Autodesk Inventor part; units mm, degrees
ref_plane "YZ Plane" through (0, 0, 0) normal (1, 0, 0) x (0, 1, 0)
ref_plane "XZ Plane" through (0, 0, 0) normal (0, 1, 0) x (-1, 0, 0)
ref_plane "XY Plane" through (0, 0, 0) normal (0, 0, 1) x (1, 0, 0)
sketch "Sketch1" plane through (0, 0, 0) normal (0, 0, 1) x (1, 0, 0)
  circle A0 centre (0, 0) radius 11.9062
  dimension "d0" = 23.8125
extrude "Extrusion1" add sketch "Sketch1" along normal blind 41.275
sketch "Sketch2" plane through (0, 0, 41.275) normal (0, 0, 1) x (1, 0, 0)
  circle A0 centre (0, 0) radius 12.7
  dimension "d3" = 25.4
extrude "Extrusion2" add sketch "Sketch2" against normal blind 23.8125
sketch "Sketch3" plane through (0, 0, 41.275) normal (0, 0, 1) x (1, 0, 0)
  line L0 (-3.6662, 6.35) -> (3.6662, 6.35)
  line L1 (3.6662, 6.35) -> (7.3323, 0)
  line L2 (7.3323, 0) -> (3.6662, -6.35)
  line L3 (3.6662, -6.35) -> (-3.6662, -6.35)
  line L4 (-3.6662, -6.35) -> (-7.3323, 0)
  line L5 (-7.3323, 0) -> (-3.6662, 6.35)
  point P0 (0, 0)
  dimension "d6" = 12.7
  dimension "d7" = 12.7
  dimension "d8" = 12.7
  dimension "d9" = 120
  dimension "d10" = 120
  dimension "d11" = 6.35
  dimension "d12" = 6.35
  dimension "d13" = 6.35
extrude "Extrusion3" cut sketch "Sketch3" against normal blind 50.8
sketch "Sketch4" plane through (0, 0, 41.275) normal (0, 0, 1) x (1, 0, 0)
  line L0 (-7.3323, 0) -> (-3.6662, 6.35)
  line L1 (-3.6662, 6.35) -> (3.6662, 6.35)
  line L2 (3.6662, 6.35) -> (7.3323, 0)
  line L3 (7.3323, 0) -> (3.6662, -6.35)
  line L4 (3.6662, -6.35) -> (-3.6662, -6.35)
  line L5 (-3.6662, -6.35) -> (-7.3323, 0)
  circle A0 centre (0, 0) radius 12.7
  line L6 (0, 12.7) -> (0, 15.875) construction
  line L7 (0, 12.7) -> (3.175, 12.7) construction
  line L8 (0, 0) -> (1.9867, 12.5436) construction
  circle A1 centre (0, 0) radius 12.7 construction
  line L9 (0, 0) -> (12.7, 0) construction
  line L10 (0, 0) -> (-1.9867, 12.5436) construction
  line L11 (0, 0) -> (12.7, 0) construction
  line L12 (0, 15.875) -> (0.7937, 15.875) construction
  line L13 (0, 15.875) -> (0.7937, 15.875) construction
  line L14 (0, 15.875) -> (-0.7937, 15.875) construction
  line L15 (0, 15.875) -> (0.7937, 15.875) construction
  line L16 (-1.9867, 12.5436) -> (-0.7937, 15.875)
  line L17 (-0.7937, 15.875) -> (0.7937, 15.875)
  line L18 (0.7937, 15.875) -> (1.9867, 12.5436)
  line L19 (-1.9867, 12.5436) -> (1.9867, 12.5436)
  line L20 (-6.35, 10.9985) -> (-7.9375, 13.7482) construction
  line L21 (-6.35, 10.9985) -> (-3.6004, 12.586) construction
  line L22 (0, 0) -> (-4.5513, 11.8565) construction
  line L23 (0, 0) -> (-7.9924, 9.8698) construction
  line L24 (-7.9375, 13.7482) -> (-7.2501, 14.145) construction
  line L25 (-7.9375, 13.7482) -> (-7.2501, 14.145) construction
  line L26 (-7.9375, 13.7482) -> (-8.6249, 13.3513) construction
  line L27 (-7.9375, 13.7482) -> (-7.2501, 14.145) construction
  line L28 (-7.9924, 9.8698) -> (-8.6249, 13.3513)
  line L29 (-8.6249, 13.3513) -> (-7.2501, 14.145)
  line L30 (-7.2501, 14.145) -> (-4.5513, 11.8565)
  line L31 (-7.9924, 9.8698) -> (-4.5513, 11.8565)
  line L32 (-10.9985, 6.35) -> (-13.7482, 7.9375) construction
  line L33 (-10.9985, 6.35) -> (-9.411, 9.0996) construction
  line L34 (0, 0) -> (-9.8698, 7.9924) construction
  line L35 (0, 0) -> (-11.8565, 4.5513) construction
  line L36 (-13.7482, 7.9375) -> (-13.3513, 8.6249) construction
  line L37 (-13.7482, 7.9375) -> (-13.3513, 8.6249) construction
  line L38 (-13.7482, 7.9375) -> (-14.145, 7.2501) construction
  line L39 (-13.7482, 7.9375) -> (-13.3513, 8.6249) construction
  line L40 (-11.8565, 4.5513) -> (-14.145, 7.2501)
  line L41 (-14.145, 7.2501) -> (-13.3513, 8.6249)
  line L42 (-13.3513, 8.6249) -> (-9.8698, 7.9924)
  line L43 (-11.8565, 4.5513) -> (-9.8698, 7.9924)
  line L44 (-12.7, 0) -> (-15.875, 0) construction
  line L45 (-12.7, 0) -> (-12.7, 3.175) construction
  line L46 (0, 0) -> (-12.5436, 1.9867) construction
  line L47 (0, 0) -> (-12.5436, -1.9867) construction
  line L48 (-15.875, 0) -> (-15.875, 0.7938) construction
  line L49 (-15.875, 0) -> (-15.875, 0.7938) construction
  line L50 (-15.875, 0) -> (-15.875, -0.7937) construction
  line L51 (-15.875, 0) -> (-15.875, 0.7938) construction
  line L52 (-12.5436, -1.9867) -> (-15.875, -0.7937)
  line L53 (-15.875, -0.7937) -> (-15.875, 0.7938)
  line L54 (-15.875, 0.7938) -> (-12.5436, 1.9867)
  line L55 (-12.5436, -1.9867) -> (-12.5436, 1.9867)
  line L56 (-10.9985, -6.35) -> (-13.7482, -7.9375) construction
  line L57 (-10.9985, -6.35) -> (-12.586, -3.6004) construction
  line L58 (0, 0) -> (-11.8565, -4.5513) construction
  line L59 (0, 0) -> (-9.8698, -7.9924) construction
  line L60 (-13.7482, -7.9375) -> (-14.145, -7.2501) construction
  line L61 (-13.7482, -7.9375) -> (-14.145, -7.2501) construction
  line L62 (-13.7482, -7.9375) -> (-13.3513, -8.6249) construction
  line L63 (-13.7482, -7.9375) -> (-14.145, -7.2501) construction
  line L64 (-9.8698, -7.9924) -> (-13.3513, -8.6249)
  line L65 (-13.3513, -8.6249) -> (-14.145, -7.2501)
  line L66 (-14.145, -7.2501) -> (-11.8565, -4.5513)
  line L67 (-9.8698, -7.9924) -> (-11.8565, -4.5513)
  line L68 (-6.35, -10.9985) -> (-7.9375, -13.7482) construction
  line L69 (-6.35, -10.9985) -> (-9.0996, -9.411) construction
  line L70 (0, 0) -> (-7.9924, -9.8698) construction
  line L71 (0, 0) -> (-4.5513, -11.8565) construction
  line L72 (-7.9375, -13.7482) -> (-8.6249, -13.3513) construction
  line L73 (-7.9375, -13.7482) -> (-8.6249, -13.3513) construction
  line L74 (-7.9375, -13.7482) -> (-7.2501, -14.145) construction
  line L75 (-7.9375, -13.7482) -> (-8.6249, -13.3513) construction
  line L76 (-4.5513, -11.8565) -> (-7.2501, -14.145)
  line L77 (-7.2501, -14.145) -> (-8.6249, -13.3513)
  line L78 (-8.6249, -13.3513) -> (-7.9924, -9.8698)
  line L79 (-4.5513, -11.8565) -> (-7.9924, -9.8698)
  line L80 (0, -12.7) -> (0, -15.875) construction
  line L81 (0, -12.7) -> (-3.175, -12.7) construction
  line L82 (0, 0) -> (-1.9867, -12.5436) construction
  line L83 (0, 0) -> (1.9867, -12.5436) construction
  line L84 (0, -15.875) -> (-0.7938, -15.875) construction
  line L85 (0, -15.875) -> (-0.7938, -15.875) construction
  line L86 (0, -15.875) -> (0.7937, -15.875) construction
  line L87 (0, -15.875) -> (-0.7938, -15.875) construction
  line L88 (1.9867, -12.5436) -> (0.7937, -15.875)
  line L89 (0.7937, -15.875) -> (-0.7938, -15.875)
  line L90 (-0.7938, -15.875) -> (-1.9867, -12.5436)
  line L91 (1.9867, -12.5436) -> (-1.9867, -12.5436)
  line L92 (6.35, -10.9985) -> (7.9375, -13.7482) construction
  line L93 (6.35, -10.9985) -> (3.6004, -12.586) construction
  line L94 (0, 0) -> (4.5513, -11.8565) construction
  line L95 (0, 0) -> (7.9924, -9.8698) construction
  line L96 (7.9375, -13.7482) -> (7.2501, -14.145) construction
  line L97 (7.9375, -13.7482) -> (7.2501, -14.145) construction
  line L98 (7.9375, -13.7482) -> (8.6249, -13.3513) construction
  line L99 (7.9375, -13.7482) -> (7.2501, -14.145) construction
  line L100 (7.9924, -9.8698) -> (8.6249, -13.3513)
  line L101 (8.6249, -13.3513) -> (7.2501, -14.145)
  line L102 (7.2501, -14.145) -> (4.5513, -11.8565)
  line L103 (7.9924, -9.8698) -> (4.5513, -11.8565)
  line L104 (10.9985, -6.35) -> (13.7482, -7.9375) construction
  line L105 (10.9985, -6.35) -> (9.411, -9.0996) construction
  line L106 (0, 0) -> (9.8698, -7.9924) construction
  line L107 (0, 0) -> (11.8565, -4.5513) construction
  line L108 (13.7482, -7.9375) -> (13.3513, -8.6249) construction
  line L109 (13.7482, -7.9375) -> (13.3513, -8.6249) construction
  line L110 (13.7482, -7.9375) -> (14.145, -7.2501) construction
  line L111 (13.7482, -7.9375) -> (13.3513, -8.6249) construction
  line L112 (11.8565, -4.5513) -> (14.145, -7.2501)
  line L113 (14.145, -7.2501) -> (13.3513, -8.6249)
  line L114 (13.3513, -8.6249) -> (9.8698, -7.9924)
  line L115 (11.8565, -4.5513) -> (9.8698, -7.9924)
  line L116 (12.7, 0) -> (15.875, 0) construction
  line L117 (12.7, 0) -> (12.7, -3.175) construction
  line L118 (0, 0) -> (12.5436, -1.9867) construction
  line L119 (0, 0) -> (12.5436, 1.9867) construction
  line L120 (15.875, 0) -> (15.875, -0.7938) construction
  line L121 (15.875, 0) -> (15.875, -0.7938) construction
  line L122 (15.875, 0) -> (15.875, 0.7937) construction
  line L123 (15.875, 0) -> (15.875, -0.7938) construction
  line L124 (12.5436, 1.9867) -> (15.875, 0.7937)
  line L125 (15.875, 0.7937) -> (15.875, -0.7938)
  line L126 (15.875, -0.7938) -> (12.5436, -1.9867)
  line L127 (12.5436, 1.9867) -> (12.5436, -1.9867)
  line L128 (10.9985, 6.35) -> (13.7482, 7.9375) construction
  line L129 (10.9985, 6.35) -> (12.586, 3.6004) construction
  line L130 (0, 0) -> (11.8565, 4.5513) construction
  line L131 (0, 0) -> (9.8698, 7.9924) construction
  line L132 (13.7482, 7.9375) -> (14.145, 7.2501) construction
  line L133 (13.7482, 7.9375) -> (14.145, 7.2501) construction
  line L134 (13.7482, 7.9375) -> (13.3513, 8.6249) construction
  line L135 (13.7482, 7.9375) -> (14.145, 7.2501) construction
  line L136 (9.8698, 7.9924) -> (13.3513, 8.6249)
  line L137 (13.3513, 8.6249) -> (14.145, 7.2501)
  line L138 (14.145, 7.2501) -> (11.8565, 4.5513)
  line L139 (9.8698, 7.9924) -> (11.8565, 4.5513)
  line L140 (6.35, 10.9985) -> (7.9375, 13.7482) construction
  line L141 (6.35, 10.9985) -> (9.0996, 9.411) construction
  line L142 (0, 0) -> (7.9924, 9.8698) construction
  line L143 (0, 0) -> (4.5513, 11.8565) construction
  line L144 (7.9375, 13.7482) -> (8.6249, 13.3513) construction
  line L145 (7.9375, 13.7482) -> (8.6249, 13.3513) construction
  line L146 (7.9375, 13.7482) -> (7.2501, 14.145) construction
  line L147 (7.9375, 13.7482) -> (8.6249, 13.3513) construction
  line L148 (4.5513, 11.8565) -> (7.2501, 14.145)
  line L149 (7.2501, 14.145) -> (8.6249, 13.3513)
  line L150 (8.6249, 13.3513) -> (7.9924, 9.8698)
  line L151 (4.5513, 11.8565) -> (7.9924, 9.8698)
  dimension "d16" = 12.7
  dimension "d17" = 0
  dimension "d18" = 3.175
  dimension "d19" = 90
  dimension "d20" = 81
  dimension "d21" = 99
  dimension "d22" = 0.7937
  dimension "d23" = 0
  dimension "d24" = 0.7937
  dimension "d25" = 180
  dimension "d28" = 360
extrude "Extrusion4" add sketch "Sketch4" against normal blind 23.8125 contours A0 L127 | A0 L124 L125 L126 | L139 A0 | A0 L136 L137 L138 | L112 L113 L114 A0 | A0 L115 | L151 A0 | A0 L148 L149 L150 | L100 L101 L102 A0 | A0 L103 | L19 A0 | A0 L16 L17 L18 | L88 L89 L90 A0 | A0 L91 | L31 A0 | A0 L28 L29 L30 | L76 L77 L78 A0 | A0 L79 | L43 A0 | A0 L40 L41 L42 | L64 L65 L66 A0 | A0 L67 | L55 A0 | A0 L52 L53 L54
properties part number "pinion"
Verification items for the finished model (mm, model axes). A direction names the side the tool comes from. Coordinates: 2 decimals unless noted, no trailing zeros. Write each loop counter-clockwise with the first axis right and the second up, starting at its lowest first coordinate (ties: lowest second). Pieces come first, ordered by that corner, then holes. Notation, with made-up numbers: M 51.25,40.25 L 106.25,40.25 A14 ccw 106.25,54.25 Z; hole C 49.25,37 d9. An arc over 180 degrees is marked long. Answer as a JSON object with one key per item and string values. Group by question number.
(1) Gauge pin test, flat ends, axial feed: pin 1 (6 mm diameter, centred on y = 9, z = 13, fed in from -X); pin 2 (6 mm diameter, centred on y = -12, z = 8, fed in from -X); pin 3 (8 mm diameter, centred on x = -1, z = 12.5, fed in from +Y). Record the tip position at first contact, or that the pin passes through.
(2) Cross-section at C-C, the plane y = 11. Record the cut outline in (x, z) (1 decimal).
(3) Release check for a two-part mould opening along X. For faces 4 (the face through (1.382, 14.233, 29.535)), 5 (the face through (-12, -2, 17.462)), 6 (the face through (8.313, 11.635, 29.535)) record: +X half, -X half, draft (parallel to the pull), parting line (faces both ways), or undercut.
(4) Cross-section at A-A, the plane z = 6.5. Record the cut outline in (x, y), and give its area (3 significant figures).
(5) Material ranges on line 1 (X direction, y = -13, z = 28.5); line 2 (Z direction, x = -13.5, y = 8) (1 decimal); line 3 (Y direction, x = -7, z = 14.5), recorded low to high.
(6) Tool access check on faces 1 (the face through (12.262, -3.305, 29.535)), 2 (the face through (-5.525, 3.131, 20.926)), 3 (the face through (-8.313, -11.635, 29.535)). Record the directions out of +Z, -Z, +X, -X, +Y, -Y that give a thin tool (end or side, any length) a straight path to the whole face; none if there is none.
Reply:
{
 "1": {"pin 1": "x = -10.28", "pin 2": "x = -7.79", "pin 3": "y = 11.91"},
 "2": {"outline": "M -8.2,17.5 L -4.6,17.5 L -4.6,0 L 4.6,0 L 4.6,17.5 L 8.2,17.5 L 8.2,41.3 L -8.2,41.3 Z"},
 "3": {"face 4": "undercut", "face 5": "draft", "face 6": "+X half"},
 "4": {"outline": "C 0,0 d23.81; hole M -7.33,0 L -3.67,-6.35 L 3.67,-6.35 L 7.33,0 L 3.67,6.35 L -3.67,6.35 Z", "area": "306 mm²"},
 "5": {"line 1": "-8.56 to -5.9, -1.82 to 1.82, 5.9 to 8.56", "line 2": "17.5 to 41.3", "line 3": "-9.63 to -0.58, 0.58 to 9.63"},
 "6": {"face 1": "+Z, -Z, +X", "face 2": "+Z, -Z", "face 3": "+Z, -Z, -X"}
}
